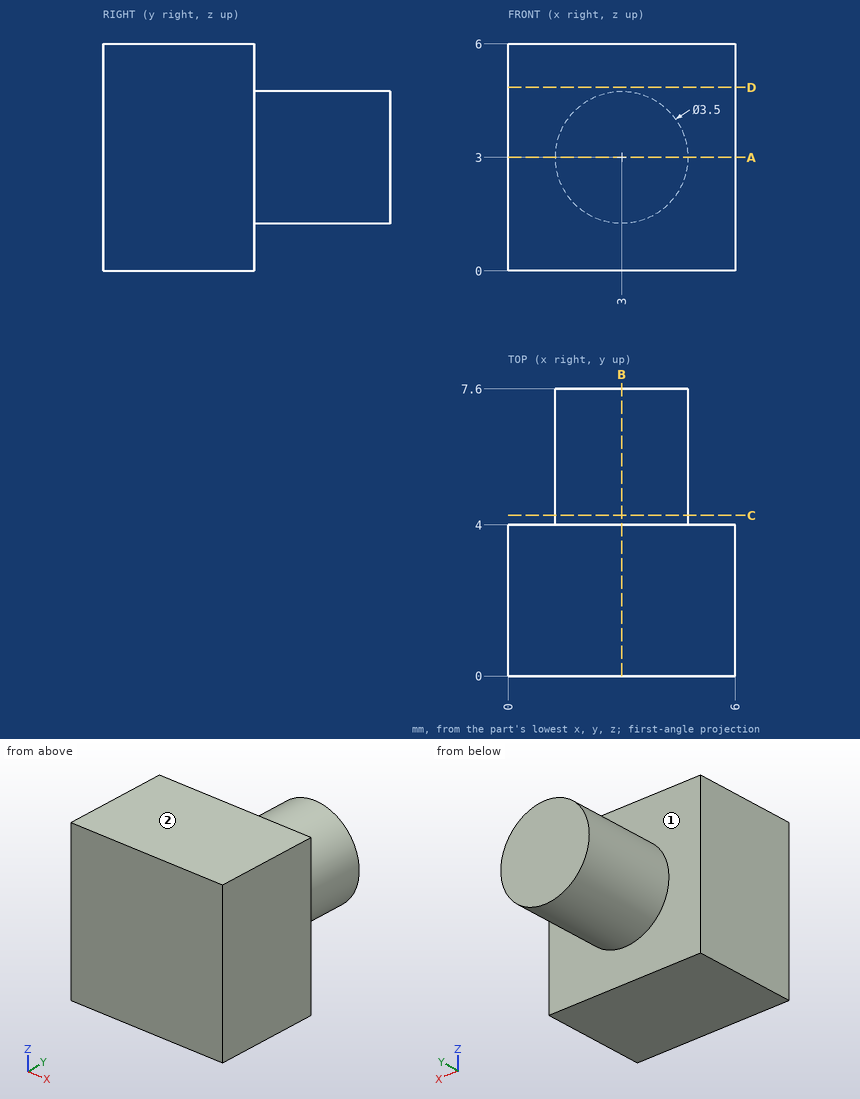
Source: three-view drawing plus pictorial views. Frame: mm from the lowest corner of the part. A direction names the side the tool comes from. Give positions to 0.01 mm unless a question says otherwise; leave off trailing zeros. Order: outer loops, then holes, each group sorted by start corner. A loop starts at its lowest first (then second) coordinate and runs counter-clockwise, first axis right, second up.
1. Section A-A on z = 3. Return the cut outline in (x, y).
Derived:
outline: (0, 0) - (6, 0) - (6, 4) - (4.75, 4) - (4.75, 7.6) - (1.25, 7.6) - (1.25, 4) - (0, 4) - close
2. Section B-B on x = 3. Return the cut outline in (y, z), and give its area (3 significant figures).
Derived:
outline: (0, 0) - (4, 0) - (4, 1.25) - (7.6, 1.25) - (7.6, 4.75) - (4, 4.75) - (4, 6) - (0, 6) - close
area: 36.6 mm2
3. Material intervals for L1, parallel to Y at x = 1.1, z = 2.6; L2, parallel to X at y = 6.25, z = 3.55; L3, parallel to X at y = 5.5, z = 2.15, sorted ascending.
Derived:
L1: y = 0 to 4
L2: x = 1.34 to 4.66
L3: x = 1.47 to 4.53
4. Section C-C on y = 4.25. Return the cut outline in (x, z).
Derived:
outline: circle Ø3.5 at (3, 3)
5. Section D-D on z = 4.85. Return the cut outline in (x, y), and give its area (3 significant figures).
Derived:
outline: (0, 0) - (6, 0) - (6, 4) - (0, 4) - close
area: 24.0 mm2
6. Pin query (flat end, axial travel): pin 1 (1 mm diameter, centred on x = 4.5, y = 3, fed in from -Z). Return the tip coordinate at first contact, or that it passes through.
Derived:
pin 1: stops at z = 0
7. Reachability of the marked faces 1 and 2 from +Z, -Z, +X, -X, +Y, -Y: full face, straight path, thin tool, end or side. Return the list, or none.
Derived:
face 1: +Y
face 2: +Z, +X, -X, +Y, -Y
